from build123d import *

# Parameters (mm, degrees)
F0_W         = 51.5
F0_H         = 26.5
F0_R         = 8
F1_DEPTH     = 11
F2_W         = 70
F2_H         = 35
F2_W_2       = 25.75
F2_H_2       = 11
F3_DEPTH     = 3
F4_SIZE      = 2
F5_T1_DEPTH  = 11
F5_T3_DEPTH  = 5.5
F5_T17_DEPTH = 8.071682988
F5_T21_DEPTH = 13.571682988
F5_T28_DEPTH = 13.571682988
F5_T32_DEPTH = 8.071682988
F5_T39_DEPTH = 13.571682988
F5_T43_DEPTH = 8.071682988
F5_T50_DEPTH = 13.571682988
F5_T54_DEPTH = 8.071682988
F5_T61_DEPTH = 8.071682988
F5_T65_DEPTH = 13.571682988
F5_T72_DEPTH = 13.571682988
F5_T76_DEPTH = 8.071682988
F5_T83_DEPTH = 13.571682988
F5_T87_DEPTH = 8.071682988
F5_T94_DEPTH = 13.571682988
F5_T98_DEPTH = 8.071682988


# Not quite as in the source:
# - a fillet or chamfer that OpenCascade refuses, or shapes differently, is made with other operations: its cross-section is extruded or revolved along the edge and cut away or added


with BuildPart() as f1:
    # F0 (on Top) → F1 (new body)
    with BuildSketch(Plane.XY):
        Rectangle(F0_W, F0_H)
        Polygon((5.5, 10.25), (22.75, 10.25), (22.75, -10.25), (-22.75, -10.25), (-22.75, 10.25), (-5.5, 10.25), align=None, mode=Mode.SUBTRACT)
        Polygon((22.75, -10.25), (22.75, 10.25), (5.5, 10.25), (5.5, 4.75), (-5.5, 4.75), (-5.5, 10.25), (-22.75, 10.25), (-22.75, -10.25), align=None)
        with Locations((-13.5, 0)):
            Circle(F0_R, mode=Mode.SUBTRACT)
        with BuildLine():
            ThreePointArc((21.5, 0), (13.5, -8), (5.5, 0))
            ThreePointArc((5.5, 0), (13.5, 8), (21.5, 0))
        make_face(mode=Mode.SUBTRACT)
    extrude(amount=F1_DEPTH)

    # F2 (on face) → F3 (join)
    with BuildSketch(Plane(origin=(0, 13.25, 0), x_dir=(-1, 0, 0), z_dir=(0, 1, 0))):
        with Locations((0, 5.5)):
            Rectangle(F2_W, F2_H)
        Polygon((25.75, 0), (0, 0), (-25.75, 0), (-25.75, 11), (0, 11), (25.75, 11), align=None, mode=Mode.SUBTRACT)
        with Locations((-12.875, 5.5)):
            Rectangle(F2_W_2, F2_H_2)
        with Locations((12.875, 5.5)):
            Rectangle(F2_W_2, F2_H_2)
    extrude(amount=F3_DEPTH)

    # F4
    f4_edges = [f1.edges().sort_by_distance(p)[0] for p in [
        (-25.75, -13.25, 5.5),
        (25.75, -13.25, 5.5),
        (0, -13.25, 11),
        (25.75, 0, 11),
        (-25.75, 0, 11),
        (25.75, 0, 0),
        (-25.75, 0, 0),
        (0, -13.25, 0),
    ]]
    chamfer(f4_edges, length=F4_SIZE)

    # F5: chamfer of 1 on 12 edges, made by hand

    # F5_s2 → F5_t1 (cut)
    with BuildSketch(Plane.YZ.offset(-5.5)):
        Polygon((3.75, 0), (4.75, 1), (4.75, 0), align=None)
        Polygon((11.25, 0), (10.25, 1), (10.25, 0), align=None)
        Polygon((3.75, 11), (4.75, 10), (4.75, 11), align=None)
        Polygon((11.25, 11), (10.25, 10), (10.25, 11), align=None)
    extrude(amount=F5_T1_DEPTH, mode=Mode.SUBTRACT)

    # F5_s4 → F5_t3 (cut)
    with BuildSketch(Plane.XZ.offset(-10.25)):
        Polygon((6.5, 0), (5.5, 1), (5.5, 0), align=None)
        Polygon((-6.5, 0), (-5.5, 1), (-5.5, 0), align=None)
        Polygon((-6.5, 11), (-5.5, 10), (-5.5, 11), align=None)
        Polygon((6.5, 11), (5.5, 10), (5.5, 11), align=None)
    extrude(amount=F5_T3_DEPTH, mode=Mode.SUBTRACT)

    # F5_s5 → F5_t6 (revolve, cut)
    with BuildSketch(Plane.XZ):
        Polygon((-4.5, 0), (-5.5, 1), (-5.5, 0), align=None)
    revolve(axis=Axis((-13.5, 0, 0), (0, 0, 1)), mode=Mode.SUBTRACT)

    # F5_s7 → F5_t8 (revolve, cut)
    with BuildSketch(Plane.XZ):
        Polygon((4.5, 0), (5.5, 1), (5.5, 0), align=None)
    revolve(axis=Axis((13.5, 0, 0), (0, 0, -1)), mode=Mode.SUBTRACT)

    # F5_s9 → F5_t10 (revolve, cut)
    with BuildSketch(Plane.XZ):
        Polygon((-4.5, 11), (-5.5, 10), (-5.5, 11), align=None)
    revolve(axis=Axis((-13.5, 0, 11), (0, 0, 1)), mode=Mode.SUBTRACT)

    # F5_s11 → F5_t12 (revolve, cut)
    with BuildSketch(Plane.XZ):
        Polygon((4.5, 11), (5.5, 10), (5.5, 11), align=None)
    revolve(axis=Axis((13.5, 0, 11), (0, 0, -1)), mode=Mode.SUBTRACT)


with BuildPart() as f5_tool15:
    # F5_s16 → F5_t17 (new body)
    with BuildSketch(Plane.XZ.offset(-10.25)):
        Polygon((6.5, 0), (5.5, 1), (5.5, 0), align=None)
    extrude(amount=F5_T17_DEPTH)

    split(bisect_by=Plane.XZ.offset(-4.75), keep=Keep.TOP)


with BuildPart() as f5_tool19:
    # F5_s20 → F5_t21 (new body)
    with BuildSketch(Plane.YZ.offset(8.071682988)):
        Polygon((3.75, 0), (4.75, 1), (4.75, 0), align=None)
    extrude(amount=-F5_T21_DEPTH)

    split(bisect_by=Plane.YZ.offset(5.5), keep=Keep.TOP)


with BuildPart() as f5_tool15_1:
    add(f5_tool15.part)

    # F5_t23: intersect F5_tool19
    add(f5_tool19.part, mode=Mode.INTERSECT)


with BuildPart() as f1_1:
    add(f1.part)

    # F5_t13: cut F5_tool15
    add(f5_tool15_1.part, mode=Mode.SUBTRACT)


with BuildPart() as f5_tool26:
    # F5_s27 → F5_t28 (new body)
    with BuildSketch(Plane.YZ.offset(5.5)):
        Polygon((3.75, 0), (4.75, 1), (4.75, 0), align=None)
    extrude(amount=-F5_T28_DEPTH)

    split(bisect_by=Plane.YZ.offset(-5.5), keep=Keep.BOTTOM)


with BuildPart() as f5_tool30:
    # F5_s31 → F5_t32 (new body)
    with BuildSketch(Plane.XZ.offset(-2.178317012)):
        Polygon((-6.5, 0), (-5.5, 1), (-5.5, 0), align=None)
    extrude(amount=-F5_T32_DEPTH)

    split(bisect_by=Plane.XZ.offset(-4.75), keep=Keep.TOP)


with BuildPart() as f5_tool26_1:
    add(f5_tool26.part)

    # F5_t34: intersect F5_tool30
    add(f5_tool30.part, mode=Mode.INTERSECT)


with BuildPart() as f1_2:
    add(f1_1.part)

    # F5_t24: cut F5_tool26
    add(f5_tool26_1.part, mode=Mode.SUBTRACT)


with BuildPart() as f5_tool37:
    # F5_s38 → F5_t39 (new body)
    with BuildSketch(Plane.YZ.offset(-5.5)):
        Polygon((11.25, 0), (10.25, 1), (10.25, 0), align=None)
    extrude(amount=F5_T39_DEPTH)

    split(bisect_by=Plane.YZ.offset(5.5), keep=Keep.TOP)


with BuildPart() as f5_tool41:
    # F5_s42 → F5_t43 (new body)
    with BuildSketch(Plane.XZ.offset(-12.821682988)):
        Polygon((6.5, 0), (5.5, 1), (5.5, 0), align=None)
    extrude(amount=F5_T43_DEPTH)

    split(bisect_by=Plane.XZ.offset(-10.25), keep=Keep.BOTTOM)


with BuildPart() as f5_tool37_1:
    add(f5_tool37.part)

    # F5_t45: intersect F5_tool41
    add(f5_tool41.part, mode=Mode.INTERSECT)


with BuildPart() as f1_3:
    add(f1_2.part)

    # F5_t35: cut F5_tool37
    add(f5_tool37_1.part, mode=Mode.SUBTRACT)


with BuildPart() as f5_tool48:
    # F5_s49 → F5_t50 (new body)
    with BuildSketch(Plane.YZ.offset(-8.071682988)):
        Polygon((11.25, 0), (10.25, 1), (10.25, 0), align=None)
    extrude(amount=F5_T50_DEPTH)

    split(bisect_by=Plane.YZ.offset(-5.5), keep=Keep.BOTTOM)


with BuildPart() as f5_tool52:
    # F5_s53 → F5_t54 (new body)
    with BuildSketch(Plane.XZ.offset(-4.75)):
        Polygon((-6.5, 0), (-5.5, 1), (-5.5, 0), align=None)
    extrude(amount=-F5_T54_DEPTH)

    split(bisect_by=Plane.XZ.offset(-10.25), keep=Keep.BOTTOM)


with BuildPart() as f5_tool48_1:
    add(f5_tool48.part)

    # F5_t56: intersect F5_tool52
    add(f5_tool52.part, mode=Mode.INTERSECT)


with BuildPart() as f1_4:
    add(f1_3.part)

    # F5_t46: cut F5_tool48
    add(f5_tool48_1.part, mode=Mode.SUBTRACT)


with BuildPart() as f5_tool59:
    # F5_s60 → F5_t61 (new body)
    with BuildSketch(Plane.XZ.offset(-10.25)):
        Polygon((6.5, 11), (5.5, 10), (5.5, 11), align=None)
    extrude(amount=F5_T61_DEPTH)

    split(bisect_by=Plane.XZ.offset(-4.75), keep=Keep.TOP)


with BuildPart() as f5_tool63:
    # F5_s64 → F5_t65 (new body)
    with BuildSketch(Plane.YZ.offset(8.071682988)):
        Polygon((3.75, 11), (4.75, 10), (4.75, 11), align=None)
    extrude(amount=-F5_T65_DEPTH)

    split(bisect_by=Plane.YZ.offset(5.5), keep=Keep.TOP)


with BuildPart() as f5_tool59_1:
    add(f5_tool59.part)

    # F5_t67: intersect F5_tool63
    add(f5_tool63.part, mode=Mode.INTERSECT)


with BuildPart() as f1_5:
    add(f1_4.part)

    # F5_t57: cut F5_tool59
    add(f5_tool59_1.part, mode=Mode.SUBTRACT)


with BuildPart() as f5_tool70:
    # F5_s71 → F5_t72 (new body)
    with BuildSketch(Plane.YZ.offset(5.5)):
        Polygon((3.75, 11), (4.75, 10), (4.75, 11), align=None)
    extrude(amount=-F5_T72_DEPTH)

    split(bisect_by=Plane.YZ.offset(-5.5), keep=Keep.BOTTOM)


with BuildPart() as f5_tool74:
    # F5_s75 → F5_t76 (new body)
    with BuildSketch(Plane.XZ.offset(-2.178317012)):
        Polygon((-6.5, 11), (-5.5, 10), (-5.5, 11), align=None)
    extrude(amount=-F5_T76_DEPTH)

    split(bisect_by=Plane.XZ.offset(-4.75), keep=Keep.TOP)


with BuildPart() as f5_tool70_1:
    add(f5_tool70.part)

    # F5_t78: intersect F5_tool74
    add(f5_tool74.part, mode=Mode.INTERSECT)


with BuildPart() as f1_6:
    add(f1_5.part)

    # F5_t68: cut F5_tool70
    add(f5_tool70_1.part, mode=Mode.SUBTRACT)


with BuildPart() as f5_tool81:
    # F5_s82 → F5_t83 (new body)
    with BuildSketch(Plane.YZ.offset(-8.071682988)):
        Polygon((11.25, 11), (10.25, 10), (10.25, 11), align=None)
    extrude(amount=F5_T83_DEPTH)

    split(bisect_by=Plane.YZ.offset(-5.5), keep=Keep.BOTTOM)


with BuildPart() as f5_tool85:
    # F5_s86 → F5_t87 (new body)
    with BuildSketch(Plane.XZ.offset(-4.75)):
        Polygon((-6.5, 11), (-5.5, 10), (-5.5, 11), align=None)
    extrude(amount=-F5_T87_DEPTH)

    split(bisect_by=Plane.XZ.offset(-10.25), keep=Keep.BOTTOM)


with BuildPart() as f5_tool81_1:
    add(f5_tool81.part)

    # F5_t89: intersect F5_tool85
    add(f5_tool85.part, mode=Mode.INTERSECT)


with BuildPart() as f1_7:
    add(f1_6.part)

    # F5_t79: cut F5_tool81
    add(f5_tool81_1.part, mode=Mode.SUBTRACT)


with BuildPart() as f5_tool92:
    # F5_s93 → F5_t94 (new body)
    with BuildSketch(Plane.YZ.offset(-5.5)):
        Polygon((11.25, 11), (10.25, 10), (10.25, 11), align=None)
    extrude(amount=F5_T94_DEPTH)

    split(bisect_by=Plane.YZ.offset(5.5), keep=Keep.TOP)


with BuildPart() as f5_tool96:
    # F5_s97 → F5_t98 (new body)
    with BuildSketch(Plane.XZ.offset(-12.821682988)):
        Polygon((6.5, 11), (5.5, 10), (5.5, 11), align=None)
    extrude(amount=F5_T98_DEPTH)

    split(bisect_by=Plane.XZ.offset(-10.25), keep=Keep.BOTTOM)


with BuildPart() as f5_tool92_1:
    add(f5_tool92.part)

    # F5_t100: intersect F5_tool96
    add(f5_tool96.part, mode=Mode.INTERSECT)


with BuildPart() as f1_8:
    add(f1_7.part)

    # F5_t90: cut F5_tool92
    add(f5_tool92_1.part, mode=Mode.SUBTRACT)


solid = f1_8.part
Read the model definition and answer for the solid it produces. Units are mm, in the model's axes. A direction names the side the tool comes from. Give positions to 0.01 mm unless a question says otherwise; leave off trailing zeros. Write each loop counter-clockwise with the first axis right and the second up, starting at its lowest first coordinate (ties: lowest second). Pieces come first, ordered by that corner, then holes. Notation, with made-up numbers: (49, -2) - (100, -2) arc R29 cw to (100, 26) - close; hole circle Ø11 at (-7.75, -22.75). An arc over 180 degrees is marked (long way). Answer in a Markdown table with one row per item. Add a question column.
Item 1: Flat-ended cylindrical pins translate along their axes: P1, Ø4, axis at x = -24, y = -4, coming from the +Z side; P2, Ø6, axis at y = 7.5, z = 5, coming from the +X side; P3, Ø10, axis at y = -7, z = 1, coming from the -X side; P4, Ø14.5, axis at x = 13.5, y = 0, coming from the +Z side. Find the tip coordinate at first contact, or state that the pin passes through.
Item 2: Determine the mould class of faces 5 (the face through (-35, 15, 5)), 6 (the face through (0, 15, -12)), 7 (the face through (-5.5, 7, 5)) for opening direction X: pulls with the +X half, pulls with the -X half, needs draft (parallel to the pull), parting line crosses it, or undercut.
Item 3: A tool of negligible diameter and unlimited length cuts with its end or side. For faces 1 (the face through (0, 1, 11)), 2 (the face through (24, -12, 1)), 3 (the face through (5.5, 8, 6)), 4 (the face through (0, 1, 0)), from which of +Z, -Z, +X, -X, +Y, -Y can it reach the whole face along a straight path? Write none if from no direction.
Item 4: Section C-C, the plane y = 12 is taken. Write down the section's boundary in (x, z), and give its area (4 significant figures).
Item 5: Section D-D, the plane x = 1 is taken. Write down the section's boundary in (y, z).
Item 6: Section B-B, the plane y = 0 is taken. Write down the section's boundary in (x, z), and give its area (4 significant figures).
Item 7: Section A-A, the plane x = -13.5 is taken. Write down the section's boundary in (y, z), and give its area (4 significant figures).
Item 8: Find the intervals of material crossed by L1, parallel to Y at x = -13.5, z = 5; L2, parallel to X at y = 10, z = 4.5; L3, parallel to Y at x = -5, z = 17.5, in increasing order.
Recorded:
| question | item | result |
|---|---|---|
| 1 | P1 | stops at z = 11 |
| 1 | P2 | stops at x = 25.75 |
| 1 | P3 | stops at x = -25.75 |
| 1 | P4 | passes through |
| 2 | face 5 | pulls with the -X half |
| 2 | face 6 | needs draft |
| 2 | face 7 | undercut |
| 3 | face 1 | +Z, +X, -X, -Y |
| 3 | face 2 | -Z, +X, -Y |
| 3 | face 3 | +Z, -Z |
| 3 | face 4 | -Z, +X, -X, -Y |
| 4 | outline | (-25.75, 2) - (-23.75, 0) - (23.75, 0) - (25.75, 2) - (25.75, 9) - (23.75, 11) - (-23.75, 11) - (-25.75, 9) - close |
| 4 | area | 558.5 mm2 |
| 5 | outline | (-13.25, 2) - (-11.25, 0) - (3.75, 0) - (4.75, 1) - (4.75, 10) - (3.75, 11) - (-11.25, 11) - (-13.25, 9) - close; (10.25, 1) - (11.25, 0) - (13.25, 0) - (13.25, -12) - (16.25, -12) - (16.25, 23) - (13.25, 23) - (13.25, 11) - (11.25, 11) - (10.25, 10) - close |
| 6 | outline | (-25.75, 2) - (-23.75, 0) - (-22.5, 0) - (-21.5, 1) - (-21.5, 10) - (-22.5, 11) - (-23.75, 11) - (-25.75, 9) - close; (-5.5, 1) - (-4.5, 0) - (4.5, 0) - (5.5, 1) - (5.5, 10) - (4.5, 11) - (-4.5, 11) - (-5.5, 10) - close; (21.5, 1) - (22.5, 0) - (23.75, 0) - (25.75, 2) - (25.75, 9) - (23.75, 11) - (22.5, 11) - (21.5, 10) - close |
| 6 | area | 202.5 mm2 |
| 7 | outline | (-13.25, 2) - (-11.25, 0) - (-9, 0) - (-8, 1) - (-8, 10) - (-9, 11) - (-11.25, 11) - (-13.25, 9) - close; (8, 1) - (9, 0) - (13.25, 0) - (13.25, -12) - (16.25, -12) - (16.25, 23) - (13.25, 23) - (13.25, 11) - (9, 11) - (8, 10) - close |
| 7 | area | 214.5 mm2 |
| 8 | L1 | y = -13.25 to -8, 8 to 16.25 |
| 8 | L2 | x = -25.75 to -5.5, 5.5 to 25.75 |
| 8 | L3 | y = 13.25 to 16.25 |
